Can you work these out from the model? Positions are in its coordinate system, mm. A direction names the side the tool comes from. Coordinates: 2 decimals unless noted, no trailing zeros. Order: outer loops, then holes, each group sorted by start corner. A loop starts at its lowest first (then second) coordinate and runs counter-clockwise, first axis right, second up. Notation, with made-up numbers: (-9.5, 87) -> (0.5, 87) arc R15 cw to (0.5, 98) -> close; hole circle Ø4 at (22.25, -14.5). An arc over 180 degrees is marked (long way). Answer in a Markdown table with one row per item.
Autodesk Inventor part; units mm, degrees
ref_plane "YZ Plane" through (0, 0, 0) normal (1, 0, 0) x (0, 1, 0)
ref_plane "XZ Plane" through (0, 0, 0) normal (0, 1, 0) x (-1, 0, 0)
ref_plane "XY Plane" through (0, 0, 0) normal (0, 0, 1) x (1, 0, 0)
sketch "スケッチ2" plane through (0, 0, 0) normal (0, 1, 0) x (-1, 0, 0)
  line L0 (0, 0) -> (136, 0)
  line L1 (136, 0) -> (136, 81)
  line L2 (136, 81) -> (0, 81)
  line L3 (0, 81) -> (0, 0)
  dimension "d2" = 81
  dimension "d3" = 136
extrude "押し出し1" add sketch "スケッチ2" along normal blind 2
sketch "スケッチ3" plane through (0, 0, 0) normal (0, 1, 0) x (-1, 0, 0)
  line L0 (5, 5) -> (131, 5)
  line L1 (131, 5) -> (131, 76)
  line L2 (131, 76) -> (5, 76)
  line L3 (5, 76) -> (5, 5)
  line L4 (136, 0) -> (136, 81)
  line L5 (136, 81) -> (0, 81)
  line L6 (132.5, 77.5) -> (126.5, 77.5)
  line L7 (126.5, 77.5) -> (126.5, 76)
  line L8 (126.5, 76) -> (132.5, 76)
  line L9 (132.5, 76) -> (132.5, 77.5)
  line L10 (131, 76) -> (132.5, 76)
  line L11 (132.5, 76) -> (132.5, 71)
  line L12 (132.5, 71) -> (131, 71)
  line L13 (131, 71) -> (131, 76)
  line L14 (131, 5) -> (132.5, 5)
  line L15 (132.5, 5) -> (132.5, 10)
  line L16 (132.5, 10) -> (131, 10)
  line L17 (131, 10) -> (131, 5)
  line L18 (132.5, 5) -> (126.5, 5)
  line L19 (126.5, 5) -> (126.5, 3.5)
  line L20 (126.5, 3.5) -> (132.5, 3.5)
  line L21 (132.5, 3.5) -> (132.5, 5)
  line L22 (5, 76) -> (3.5, 76)
  line L23 (3.5, 76) -> (3.5, 71)
  line L24 (3.5, 71) -> (5, 71)
  line L25 (5, 71) -> (5, 76)
  line L26 (3.5, 76) -> (9.5, 76)
  line L27 (9.5, 76) -> (9.5, 77.5)
  line L28 (9.5, 77.5) -> (3.5, 77.5)
  line L29 (3.5, 77.5) -> (3.5, 76)
  line L30 (5, 5) -> (3.5, 5)
  line L31 (3.5, 5) -> (3.5, 10)
  line L32 (3.5, 10) -> (5, 10)
  line L33 (5, 10) -> (5, 5)
  line L34 (3.5, 5) -> (9.5, 5)
  line L35 (9.5, 5) -> (9.5, 3.5)
  line L36 (9.5, 3.5) -> (3.5, 3.5)
  line L37 (3.5, 3.5) -> (3.5, 5)
  point P0 (0, 0)
  dimension "d6" = 126
  dimension "d7" = 71
  dimension "d8" = 5
  dimension "d9" = 5
  dimension "d10" = 1.5
  dimension "d11" = 1.5
  dimension "d12" = 5
  dimension "d13" = 6
  dimension "d14" = 0
  dimension "d17" = 1.5
  dimension "d18" = 1.5
  dimension "d19" = 6
  dimension "d20" = 5
  dimension "d21" = 5
  dimension "d22" = 1.5
  dimension "d23" = 1.5
  dimension "d24" = 6
  dimension "d25" = 6
  dimension "d26" = 1.5
  dimension "d27" = 1.5
  dimension "d28" = 5
extrude "押し出し2" add sketch "スケッチ3" against normal blind 9.01 contours L30 L31 L32 L3 | L0 L35 L36 L37 L30 | L0 L14 L21 L20 L19 | L24 L23 L22 L3 | L1 L16 L15 L14 | L22 L29 L28 L27 L2 | L1 L8 L11 L12 | L7 L6 L9 L8 L2
sketch "スケッチ5" plane through (0, 0, 0) normal (0, 1, 0) x (-1, 0, 0)
  line L0 (131, 76) -> (5, 76)
  line L1 (5, 76) -> (5, 5)
  line L2 (5, 5) -> (131, 5)
  line L3 (131, 5) -> (131, 76)
  line L4 (0, 81) -> (0, 0)
  line L5 (131, 76) -> (5, 76)
  line L6 (5, 76) -> (5, 77.5)
  line L7 (5, 77.5) -> (131, 77.5)
  line L8 (131, 77.5) -> (131, 76)
  line L9 (131, 5) -> (5, 5)
  line L10 (5, 5) -> (5, 3.5)
  line L11 (5, 3.5) -> (131, 3.5)
  line L12 (131, 3.5) -> (131, 5)
  line L13 (131, 77.5) -> (132.5, 77.5)
  line L14 (132.5, 77.5) -> (132.5, 3.5)
  line L15 (132.5, 3.5) -> (131, 3.5)
  line L16 (131, 3.5) -> (131, 77.5)
  line L17 (5, 77.5) -> (3.5, 77.5)
  line L18 (3.5, 77.5) -> (3.5, 3.5)
  line L19 (3.5, 3.5) -> (5, 3.5)
  line L20 (5, 3.5) -> (5, 77.5)
  dimension "d34" = 126
  dimension "d35" = 71
  dimension "d36" = 5
  dimension "d37" = 5
  dimension "d38" = 1.5
  dimension "d39" = 1.5
  dimension "d40" = 1.5
  dimension "d41" = 1.5
  dimension "d42" = 1.5
  dimension "d43" = 1.5
extrude "押し出し4" add sketch "スケッチ5" against normal blind 2 contours L8 L13 L14 L15 L12 L3 | L0 L6 L7 L8 | L1 L10 L19 L18 L17 L6 | L12 L11 L10 L2
sketch "スケッチ7" plane through (0, 0, 0) normal (0, 1, 0) x (-1, 0, 0)
  line L0 (9, 73.5) -> (127, 73.5)
  line L1 (127, 73.5) -> (127, 7.5)
  line L2 (127, 7.5) -> (9, 7.5)
  line L3 (9, 7.5) -> (9, 73.5)
  line L4 (136, 0) -> (136, 81)
  line L5 (136, 81) -> (0, 81)
  point P0 (0, 0)
  dimension "d50" = 66
  dimension "d51" = 118
  dimension "d52" = 9
  dimension "d53" = 7.5
extrude "押し出し6" cut sketch "スケッチ7" along normal up to next
sketch "スケッチ9" plane through (-132.5, 0, 77.5) normal (0, 0, 1) x (1, 0, 0)
  line L0 (129, 0) -> (129, -9.01)
  line L1 (0, 0) -> (129, 0)
  line L2 (0, 0) -> (129, 0)
  line L3 (129, 0) -> (129, -1)
  line L4 (129, -1) -> (0, -1)
  line L5 (0, -1) -> (0, 0)
  point P0 (132.5, 0)
  dimension "d62" = 1
extrude "押し出し8" add sketch "スケッチ9" along normal blind 1.5
sketch "スケッチ10" plane through (-3.5, 0, 3.5) normal (0, 0, -1) x (-1, 0, 0)
  line L0 (129, 0) -> (129, -9.01)
  line L1 (0, 0) -> (129, 0)
  line L2 (129, 0) -> (129, -1)
  line L3 (129, -1) -> (0, -1)
  line L4 (0, -1) -> (0, 0)
  point P0 (-3.5, 0)
  dimension "d65" = 1
extrude "押し出し9" add sketch "スケッチ10" along normal blind 1.5
sketch "スケッチ11" plane through (-3.5, -9.01, 10) normal (1, 0, 0) x (0, 0, -1)
  line L0 (-69, 9.01) -> (8, 9.01)
  line L1 (8, 9.01) -> (8, 8.01)
  line L2 (8, 8.01) -> (-69, 8.01)
  line L3 (-69, 8.01) -> (-69, 9.01)
  point P0 (10, 9.01)
extrude "押し出し10" add sketch "スケッチ11" along normal blind 1.5
sketch "スケッチ12" plane through (-132.5, -9.01, 3.5) normal (-1, 0, 0) x (0, 0, 1)
  line L0 (-1.5, 9.01) -> (75.5, 9.01)
  line L1 (75.5, 9.01) -> (75.5, 8.01)
  line L2 (75.5, 8.01) -> (-1.5, 8.01)
  line L3 (-1.5, 8.01) -> (-1.5, 9.01)
  point P0 (-3.5, 9.01)
extrude "押し出し11" add sketch "スケッチ12" along normal blind 1.5
sketch "スケッチ13" plane through (0, 2, 0) normal (0, 1, 0) x (1, 0, 0)
  line L0 (-127, -7.5) -> (-9, -7.5)
  line L1 (-9, -7.5) -> (-9, -73.5)
  line L2 (-9, -73.5) -> (-127, -73.5)
  line L3 (-9, -73.5) -> (-127, -73.5)
  line L4 (-127, -73.5) -> (-127, -7.5)
  line L5 (-127, -7.5) -> (-9, -7.5)
  line L6 (-122, -7.5) -> (-114, -7.5)
  line L7 (-114, -7.5) -> (-114, -15.5)
  line L8 (-114, -15.5) -> (-122, -15.5)
  line L9 (-122, -15.5) -> (-122, -7.5)
  line L10 (-122, -73.5) -> (-114, -73.5)
  line L11 (-114, -73.5) -> (-114, -65.5)
  line L12 (-114, -65.5) -> (-122, -65.5)
  line L13 (-122, -65.5) -> (-122, -73.5)
  line L14 (-14, -7.5) -> (-22, -7.5)
  line L15 (-22, -7.5) -> (-22, -15.5)
  line L16 (-22, -15.5) -> (-14, -15.5)
  line L17 (-14, -15.5) -> (-14, -7.5)
  line L18 (-14, -73.5) -> (-22, -73.5)
  line L19 (-22, -73.5) -> (-22, -65.5)
  line L20 (-22, -65.5) -> (-14, -65.5)
  line L21 (-14, -65.5) -> (-14, -73.5)
  circle A0 centre (-118, -12.5) radius 1.25
  circle A1 centre (-118, -68.5) radius 1.25
  circle A2 centre (-18, -12.5) radius 1.25
  circle A3 centre (-18, -68.5) radius 1.25
  point P0 (-44.5213, -7.5)
  point P1 (-44.5213, -73.5)
  point P2 (-91.4787, -7.5)
  point P3 (-91.4787, -73.5)
  dimension "d72" = 8
  dimension "d73" = 8
  dimension "d74" = 8
  dimension "d75" = 8
  dimension "d76" = 8
  dimension "d77" = 8
  dimension "d78" = 8
  dimension "d79" = 8
  dimension "d80" = 5
  dimension "d81" = 5
  dimension "d82" = 5
  dimension "d83" = 5
  dimension "d84" = 2.5
  dimension "d85" = 2.5
  dimension "d86" = 2.5
  dimension "d87" = 2.5
  dimension "d88" = 4
  dimension "d89" = 3
  dimension "d90" = 3
  dimension "d91" = 4
  dimension "d92" = 4
  dimension "d93" = 5
  dimension "d94" = 4
  dimension "d95" = 5
extrude "押し出し12" add sketch "スケッチ13" against normal blind 2 contours L0 L7 L8 L9 | L13 L12 L11 L2 | L0 L17 L16 L15 | L19 L20 L21 L2
fillet "フィレット1" radius 3 8 edges at (-14, 1, 65.5) (-22, 1, 65.5) (-114, 1, 65.5) (-122, 1, 65.5) (-114, 1, 15.5) (-122, 1, 15.5) (-14, 1, 15.5) (-22, 1, 15.5)
fillet "フィレット2" radius 1.5 8 edges at (0, 1, 81) (0, 1, 0) (-136, 1, 0) (-136, 1, 81) (-134, -0.5, 79) (-134, -0.5, 2) (-2, -0.5, 2) (-2, -0.5, 79)
sketch "スケッチ15" plane through (0, -2, 0) normal (0, -1, 0) x (1, 0, 0)
  line L0 (-101.5, 77.5) -> (-101.5, 76)
  line L1 (-126.5, 76) -> (-9.5, 76)
  line L2 (-9.5, 77.5) -> (-126.5, 77.5)
  line L3 (-93, 77.5) -> (-43, 77.5)
  line L4 (-43, 77.5) -> (-43, 76)
  line L5 (-43, 76) -> (-93, 76)
  line L6 (-93, 76) -> (-93, 77.5)
  point P0 (-34.5, 76)
  point P1 (-34.5, 77.5)
  point P2 (0, 0)
  dimension "d107" = 50
  dimension "d108" = 8.5
extrude "押し出し14" [suppressed]
fillet "フィレット4" radius 2 8 edges at (-131.75, -9.01, 71) (-131.75, -9.01, 10) (-126.5, -9.01, 4.25) (-4.25, -9.01, 71) (-4.25, -9.01, 10) (-9.5, -9.01, 4.25) (-126.5, -9.01, 76.75) (-9.5, -9.01, 76.75)
equation "\"d52\" = 0.5 * d3 - 0.5 * d51"
equation "\"d53\" = 0.5 * d2 - 0.5 * d50"
properties part number "lower"
(1) On a 3-axis mill with a long thin cutter (end or side, diameter ignored), from which of +Z, -Z, +X, -X, +Y, -Y can I reach the whole of each face in a straight line? I mean faces 5 (the flat face through (-68.3, -1.7, 3.5)), 6 (the flat face through (-68.3, -1.7, 77.5)), 7 (the cylindrical face through (-121.14, 0.99, 66.4)), 8 (the flat face through (-68, 0, 75)). Say none if no direction works.
Response values:
| item | result |
|---|---|
| face 5 | -Z, +X, -X, -Y |
| face 6 | +Z, +X, -X, -Y |
| face 7 | +Y, -Y |
| face 8 | -Y |
(2) Suppose I cut it at A-A (y = -5.25). Please give me the cut outline in (x, z), and give its area (3 significant figures).
Response values:
| item | result |
|---|---|
| outline | (-132.5, 3.5) -> (-126.5, 3.5) -> (-126.5, 5) -> (-131, 5) -> (-131, 10) -> (-132.5, 10) -> close; (-132.5, 71) -> (-131, 71) -> (-131, 76) -> (-126.5, 76) -> (-126.5, 77.5) -> (-132.5, 77.5) -> close; (-9.5, 3.5) -> (-3.5, 3.5) -> (-3.5, 10) -> (-5, 10) -> (-5, 5) -> (-9.5, 5) -> close; (-9.5, 76) -> (-5, 76) -> (-5, 71) -> (-3.5, 71) -> (-3.5, 77.5) -> (-9.5, 77.5) -> close |
| area | 66.0 mm2 |
(3) Will these pins go through, and if not, where does the flat tip stop? pin 1 Ø0.8 at (y, z) = (-0.5, 49) entering from -X; pin 2 Ø0.8 at (x, z) = (-4, 41) entering from -Y; pin 3 Ø1.2 at (x, y) = (-4, -3.5) entering from -Z.
Response values:
| item | result |
|---|---|
| pin 1 | x = -134 |
| pin 2 | y = -2 |
| pin 3 | z = 3.5 |
(4) Suppose I cut it at B-B (z = 40). Please give me the cut outline in (x, y).
Response values:
| item | result |
|---|---|
| outline | (-136, 0) -> (-134, 0) -> (-134, -1) -> (-132.5, -1) -> (-132.5, -2) -> (-131, -2) -> (-131, 0) -> (-127, 0) -> (-127, 2) -> (-136, 2) -> close; (-9, 0) -> (-5, 0) -> (-5, -2) -> (-3.5, -2) -> (-3.5, -1) -> (-2, -1) -> (-2, 0) -> (0, 0) -> (0, 2) -> (-9, 2) -> close |
(5) We'd pull the mould along X, two halves only. Please class faces 1 (the flat face through (-3.5, -1.7, 40.3)), 2 (the flat face through (-68, -1, 76)), 3 (the cylindrical face through (-114.86, 0.99, 14.6)), 4 (the flat face through (-4.6, -9.01, 5.3)): +X half, -X half, draft (parallel to the pull), parting line (faces both ways), or undercut.
Response values:
| item | result |
|---|---|
| face 1 | +X half |
| face 2 | undercut |
| face 3 | undercut |
| face 4 | draft |
(6) Suppose I cut it at C-C (x = -12). Please give me the cut outline in (y, z), and give its area (3 significant figures).
Response values:
| item | result |
|---|---|
| outline | (-2, 3.5) -> (-1, 3.5) -> (-1, 2) -> (0, 2) -> (0, 0) -> (2, 0) -> (2, 7.5) -> (0, 7.5) -> (0, 5) -> (-2, 5) -> close; (-2, 76) -> (0, 76) -> (0, 73.5) -> (2, 73.5) -> (2, 81) -> (0, 81) -> (0, 79) -> (-1, 79) -> (-1, 77.5) -> (-2, 77.5) -> close |
| area | 39.0 mm2 |
(7) I need wall thicknesses on line 1 (X direction, y = 0.6, z = 68.5); line 2 (Z direction, x = -18, y = 1.25); line 3 (Z direction, x = -128, y = -0.75). Which ranges of each line are inside material? Lowest first, please. Write a range as [from, to].
Response values:
| item | result |
|---|---|
| line 1 | [-136, -127], [-122, -119.25], [-116.75, -114], [-22, -19.25], [-16.75, -14], [-9, 0] |
| line 2 | [0, 11.25], [13.75, 15.5], [65.5, 67.25], [69.75, 81] |
| line 3 | [2, 5], [76, 79] |
